```python
from build123d import *

# Parameters (mm, degrees)
SKETCH1_R                = 1.905
SKETCH1_R_2              = 1.27
BOSS_EXTRUDE1_DEPTH      = 44.45
BOSS_EXTRUDE3_DEPTH      = 0.762
BOSS_EXTRUDE3_DEPTH_BACK = 4.572
SKETCH4_R                = 1.27
CUT_EXTRUDE2_DEPTH       = 46.99
SKETCH5_W                = 3.302
SKETCH5_H                = 0.381
CUT_EXTRUDE3_DEPTH       = 1.016
SKETCH6_R                = 0.381
CUT_EXTRUDE4_DEPTH       = 5.588
SKETCH8_R                = 0.254
CUT_EXTRUDE5_DEPTH       = 1.27


with BuildPart() as part:
    # Sketch1 → Boss-Extrude1 (new body)
    with BuildSketch(Plane(origin=(0, 0, 0), x_dir=(0, 0, -1), z_dir=(1, 0, 0))):
        with Locations((-37.290755903, 15.049483632)):
            Circle(SKETCH1_R)
        with Locations((-37.290755903, 15.049483632)):
            Circle(SKETCH1_R_2, mode=Mode.SUBTRACT)
    extrude(amount=BOSS_EXTRUDE1_DEPTH)

    # Sketch2 → Boss-Extrude3 (add, two sides: drawn at the far end of the back side and taken through both)
    with BuildSketch(Plane.XY.offset(39.195755903).offset(-BOSS_EXTRUDE3_DEPTH_BACK)):
        Polygon((32.385, 15.120134353), (33.02, 15.120134353), (33.02, 12.199134353), (25.4, 12.199134353), (25.4, 15.120134353), (26.035, 15.120134353), (31.75, 15.120134353), align=None)
    extrude(amount=BOSS_EXTRUDE3_DEPTH + BOSS_EXTRUDE3_DEPTH_BACK)

    # Sketch4 → Cut-Extrude2 (cut)
    with BuildSketch(Plane.ZY):
        with Locations(Location((37.290755903, 15.049483632, 0), (0, 0, 180))):
            Circle(SKETCH4_R)
    extrude(amount=-CUT_EXTRUDE2_DEPTH, mode=Mode.SUBTRACT)

    # Sketch5 → Cut-Extrude3 (cut)
    with BuildSketch(Plane.XY.offset(39.195755903)):
        with Locations((29.21, 15.310634353)):
            Rectangle(SKETCH5_W, SKETCH5_H)
    extrude(amount=-CUT_EXTRUDE3_DEPTH, mode=Mode.SUBTRACT)

    # Sketch6 → Cut-Extrude4 (cut)
    with BuildSketch(Plane.XY.offset(39.957755903)):
        with Locations((29.21, 12.789684353)):
            Circle(SKETCH6_R)
    extrude(amount=-CUT_EXTRUDE4_DEPTH, mode=Mode.SUBTRACT)

    # Sketch8 → Cut-Extrude5 (cut)
    with BuildSketch(Plane(origin=(0, 15.120134353, 0), x_dir=(1, 0, 0), z_dir=(0, 1, 0))):
        with Locations(Location((29.21, -39.576755903, 0), (0, 0, 270))):
            Circle(SKETCH8_R)
    extrude(amount=-CUT_EXTRUDE5_DEPTH, mode=Mode.SUBTRACT)


solid = part.part
```
The listing builds one solid part. Answer for the finished solid, in the listing's coordinates (mm). A direction names the side the tool comes from. Give positions to 0.01 mm unless a question says otherwise; leave off trailing zeros. Order: outer loops, then holes, each group sorted by start corner. A loop starts at its lowest first (then second) coordinate and runs counter-clockwise, first axis right, second up. Notation, with made-up numbers: M 61.5,-14 L 110.5,-14 A23 ccw 110.5,3 Z; hole C 85.25,22 d2. An arc over 180 degrees is marked long. Put each result on its own line as item: value. Start each with the question number.
Item 1: The part is cut by section C-C, the plane x = 18. Determine the outline of the cut face in (y, z) (3 decimals), and give its area (3 significant figures).
Item 2: For a pull along Z with two mould halves and no side action, classify faces 4 (the face through (29, 12.199, 37)), 5 (the face through (21.91, 16.31, 37.46)), 6 (the face through (29, 14, 34.624)) as +Z half, -Z half, draft (parallel to the pull), parting line (faces both ways), or undercut.
Item 3: The part is cut by section A-A, the plane z = 36.55. Determine the outline of the cut face in (x, y), and give its area (3 significant figures).
Item 4: Find the intervals of material crossed by line 1 along Y through (x, z) = (29.21, 38.6); line 2 along Z through (x, y) = (18, 14.9); line 3 along Y through (x, z) = (27, 38.15), in increasing order.
Item 5: The part is cut by section B-B, the plane x = 26. Determine the outline of the cut face in (y, z) (3 decimals), and give its area (3 significant figures).
Item 6: A flat-ended cylindrical pin translates along its axis: P1, Ø1, axis at x = 9, z = 38, coming from the +Y side. Find the tip coordinate at first contact, or state that the pin passes through.
Item 7: Which of the six approach directions +Z, -Z, +X, -X, +Y, -Y give full straight-line access (tool end or side, diameter ignored) to faces 1 (the face through (29, 15.12, 39)), 2 (the face through (25.4, 13, 37)), 3 (the face through (33.02, 13, 37))?
Answer key:
1. outline: C 15.049,37.291 d3.81; hole C 15.049,37.291 d2.54
1. area: 6.33 mm²
2. face 4: draft
2. face 5: undercut
2. face 6: -Z half
3. outline: M 0,13.29 L 25.4,13.29 L 25.4,12.2 L 33.02,12.2 L 33.02,13.29 L 44.45,13.29 L 44.45,14.02 L 0,14.02 Z; M 0,16.08 L 44.45,16.08 L 44.45,16.8 L 0,16.8 Z; hole C 29.21,12.79 d0.76
3. area: 72.2 mm²
4. line 1: y = 12.2 to 12.41, 13.17 to 15.12, 15.5 to 16.43
4. line 2: z = 35.39 to 36.03, 38.55 to 39.19
4. line 3: y = 12.2 to 14.11, 15.98 to 16.75
5. outline: M 12.199,34.624 L 15.12,34.624 L 15.12,35.387 A1.905 ccw 15.12,39.194 L 15.12,39.958 L 12.199,39.958 Z; hole C 15.049,37.291 d2.54
5. area: 15.9 mm²
6. P1: stops at y = 16.94
7. face 1: +Z
7. face 2: -X, -Y
7. face 3: +X, -Y
